```python
from build123d import *

# Parameters (mm, degrees)
CUT_EXTRUDE3_DEPTH      = 45
CUT_EXTRUDE3_DEPTH_BACK = 20
CUT_EXTRUDE5_START      = -5
CUT_EXTRUDE5_DEPTH      = 5
BOSS_EXTRUDE2_DEPTH     = 5
SKETCH14_R              = 1
BOSS_EXTRUDE3_DEPTH     = 3
BOSS_EXTRUDE4_START     = 3
SKETCH15_R              = 1
BOSS_EXTRUDE4_DEPTH     = 3
CUT_EXTRUDE6_DEPTH      = 22


with BuildPart() as part:
    # Sketch1 → Revolve1 (revolve)
    with BuildSketch(Plane.XY, mode=Mode.PRIVATE) as revolve1_sk:
        with BuildLine():
            Line((20.9, 0), (23.871591838, 0))
            Line((23.871591838, 0), (23.871591838, 4))
            Line((23.871591838, 4), (22.9, 4.236662843))
            Line((22.9, 4.236662843), (22.9, 11.874576818))
            ThreePointArc((22.9, 11.874576818), (23.83692213, 16.100759435), (26.472123903, 19.535021249))
            Line((26.472123903, 19.535021249), (26.427876097, 19.497892931))
            ThreePointArc((26.427876097, 19.497892931), (29.06307787, 22.932154745), (30, 27.158337362))
            Line((30, 27.158337362), (30, 50))
            ThreePointArc((30, 50), (28.828427125, 52.828427125), (26, 54))
            Line((26, 54), (0, 54))
            Line((0, 54), (0, 15))
            Line((0, 15), (19.9, 15))
            ThreePointArc((19.9, 15), (20.607106781, 14.707106781), (20.9, 14))
            Line((20.9, 14), (20.9, 0))
        make_face()
    revolve(revolve1_sk.sketch.rotate(Axis((0, 0, 0), (0, 1, 0)), 90), axis=Axis((0, 0, 0), (0, 1, 0)))

    # Sketch11 → Cut-Extrude3 (cut, two sides: drawn at the far end of the back side and taken through both)
    with BuildSketch(Plane(origin=(0, 17, 0), x_dir=(1, 0, 0), z_dir=(0, 1, 0)).offset(-CUT_EXTRUDE3_DEPTH_BACK)):
        with BuildLine():
            Line((-17.5, 0), (17.5, 0))
            ThreePointArc((17.5, 0), (0, 17.5), (-17.5, 0))
        make_face()
    extrude(amount=CUT_EXTRUDE3_DEPTH + CUT_EXTRUDE3_DEPTH_BACK, mode=Mode.SUBTRACT)

    # Sketch9 → Cut-Extrude5 (cut)
    with BuildSketch(Plane(origin=(0, 50, 0), x_dir=(-1, 0, 0), z_dir=(0, -1, 0)).offset(CUT_EXTRUDE5_START)):
        with BuildLine():
            Line((-30, 0), (30, 0))
            ThreePointArc((30, 0), (0, 30), (-30, 0))
        make_face()
    extrude(amount=CUT_EXTRUDE5_DEPTH, mode=Mode.SUBTRACT)

    # Sketch13 → Boss-Extrude2 (add)
    with BuildSketch(Plane(origin=(0, 0, 0), x_dir=(-1, 0, 0), z_dir=(0, 0, -1))):
        with BuildLine():
            Line((22.5, 53.5), (26.5, 53.5))
            ThreePointArc((26.5, 53.5), (26.853553391, 53.353553391), (27, 53))
            Line((27, 53), (27, 51))
            ThreePointArc((27, 51), (26.853553391, 50.646446609), (26.5, 50.5))
            Line((26.5, 50.5), (22.5, 50.5))
            ThreePointArc((22.5, 50.5), (22.146446609, 50.646446609), (22, 51))
            Line((22, 51), (22, 53))
            ThreePointArc((22, 53), (22.146446609, 53.353553391), (22.5, 53.5))
        make_face()
        with BuildLine():
            Line((-26.5, 53.5), (-22.5, 53.5))
            ThreePointArc((-22.5, 53.5), (-22.146446609, 53.353553391), (-22, 53))
            Line((-22, 53), (-22, 51))
            ThreePointArc((-22, 51), (-22.146446609, 50.646446609), (-22.5, 50.5))
            Line((-22.5, 50.5), (-26.5, 50.5))
            ThreePointArc((-26.5, 50.5), (-26.853553391, 50.646446609), (-27, 51))
            Line((-27, 51), (-27, 53))
            ThreePointArc((-27, 53), (-26.853553391, 53.353553391), (-26.5, 53.5))
        make_face()
    extrude(amount=BOSS_EXTRUDE2_DEPTH)

    # Sketch14 → Boss-Extrude3 (add)
    with BuildSketch(Plane.ZY.offset(-22)):
        with Locations(Location((-3, 52, 0), (0, 0, 270))):
            Circle(SKETCH14_R)
    extrude(amount=BOSS_EXTRUDE3_DEPTH)

    # Sketch15 → Boss-Extrude4 (add)
    with BuildSketch(Plane(origin=(-22, 0, 0), x_dir=(0, 0, -1), z_dir=(1, 0, 0)).offset(BOSS_EXTRUDE4_START)):
        with Locations(Location((3, 52, 0), (0, 0, 270))):
            Circle(SKETCH15_R)
    extrude(amount=-BOSS_EXTRUDE4_DEPTH)

    # Sketch16 → Cut-Extrude6 (cut)
    with BuildSketch(Plane(origin=(0, 50, 0), x_dir=(-1, 0, 0), z_dir=(0, -1, 0))):
        with BuildLine():
            Line((28.470379344, -4), (-28.470379344, -4))
            ThreePointArc((-28.470379344, -4), (0, -28.75), (28.470379344, -4))
        make_face()
    extrude(amount=CUT_EXTRUDE6_DEPTH, mode=Mode.SUBTRACT)


solid = part.part
```
Geometry check sheet. Reference: the model listing, model coordinates, mm. A direction names the side the tool comes from. Coordinates: 2 decimals unless noted, no trailing zeros. Write each loop counter-clockwise with the first axis right and the second up, starting at its lowest first coordinate (ties: lowest second). Pieces come first, ordered by that corner, then holes. Notation, with made-up numbers: (89.25, -2) -> (126.25, -2) arc R19 ccw to (126.25, 23) -> close; hole circle Ø3 at (40.5, 8). An arc over 180 degrees is marked (long way). Use CSV: the item, a comma, the result in double quotes. Start each with the question number.
Item 1: Set-up check for faces 4 (the flat face through (-22, 52, -4.4)), 5 (the flat face through (-27, 52, -2)), 6 (the cylindrical face through (-23.67, 2.03, 3.11)), 7 (the flat face through (-25, 50.5, -2)), 8 (the cylindrical face through (20.521, 52.737, -2.324)): record each of +Z, -Z, +X, -X, +Y, -Y from which the full face is reachable in a straight line by a thin tool's end or side.
Item 2: Cross-section at C-C, the plane y = 9.5. Record the cut outline in (x, z).
Item 3: Mould release check, pull along Y, two halves, no side actions. Record for faces 1 (the flat face through (27, 52, -2)), 2 (the flat face through (0, 28, 13)), 3 (the flat face through (0, 15, 4)): released by +Y, released by -Y, zero draft, split by the parting line, or undercut.
Item 4: Thickness scan on line 1 (Z direction, x = 0.5, y = 32); line 2 (X direction, y = 9, z = 0); line 3 (X direction, y = 3.5, z = 0). Record the ranges inside material, lowest first.
Item 5: Cross-section at B-B, the plane y = 41.5. Record the cut outline in (x, z).
Item 6: Depth check by flat-ended pin: pin 1 Ø12 at (y, z) = (13, -19) entering from +X; pin 2 Ø12 at (y, z) = (25.5, 20) entering from +X; pin 3 Ø2 at (y, z) = (14, 0.5) entering from -X. Enter the tip coordinate at first touch or a pass-through.
Item 7: Cross-section at A-A, the plane x = 0. State how many separate pieces and enclosed holes the cut face has, plus the area to 3 significant figures.
Answers:
1,face 4,"-Z"
1,face 5,"-Z, -X, +Y"
1,face 6,"-Y"
1,face 7,"-Z, +X, -X"
1,face 8,"none"
2,outline,"circle Ø45.8 at (0, 0); hole circle Ø41.8 at (0, 0)"
3,face 1,"zero draft"
3,face 2,"undercut"
3,face 3,"released by -Y"
4,line 1,"-30 to -17.49, 0 to 4, 28.75 to 30"
4,line 2,"-22.9 to -20.9, 20.9 to 22.9"
4,line 3,"-23.87 to -20.9, 20.9 to 23.87"
5,outline,"circle Ø60 at (0, 0); hole (-28.47, 4) -> (28.47, 4) arc R28.75 ccw to start; hole (-17.5, 0) arc R17.5 ccw to (17.5, 0) -> close"
6,pin 1,"x = 19.51"
6,pin 2,"x = 26.46"
6,pin 3,"x = -23.4"
7,separate pieces,"2"
7,enclosed holes,"1"
7,area,"1,060 mm^2"
